The listing builds one solid part. Answer for the finished solid, in the listing's coordinates (mm). Face numbers are marked on the shaded views. A direction names the side the tool comes from. Round coordinates to 2 decimals unless told otherwise and drop trailing zeros. Order: outer loops, then holes, each group sorted by start corner. A loop starts at its lowest first (then second) coordinate and runs counter-clockwise, first axis right, second up. Notation, with made-up numbers: (-30.75, 9.5) - (-24.75, 9.5) arc R27 cw to (-24.75, 26.5) - close; hole circle Ø10 at (73, 26.5). An arc over 180 degrees is marked (long way). Write item = value, one per line.
Autodesk Fusion 360 part; units mm, degrees
sketch "Sketch1" plane through (0, 0, 0) normal (0, 0, 1) x (1, 0, 0)
  circle A0 centre (0, 0) radius 17.5
  dimension "d1" = 35
ref_plane "WorkPlane1" through (0, 0, 18) normal (0, 0, 1) x (1, 0, 0)
sketch "Sketch2" plane through (0, 0, 18) normal (0, 0, 1) x (1, 0, 0)
  circle A0 centre (0, 0) radius 17.5
  dimension "d3" = 35
ref_plane "WorkPlane2" through (0, 0, 9) normal (0, 0, 1) x (1, 0, 0)
sketch "Sketch3" plane through (0, 0, 9) normal (0, 0, 1) x (1, 0, 0)
  circle A0 centre (0, 0) radius 12.5
  dimension "d5" = 25
loft "Loft1" add profiles "Sketch2", "Sketch3" section 1 section 2
loft "Loft2" add profiles "Sketch1" section 1 section 2 face at (-3.3879, -0.621, 9)
extrude "Extrude1" add 1 faces at (4.4225, -5.9212, 18) along direction (0, 0, 1) blind 3
extrude "Extrude2" add 1 faces at (4.4225, -5.9212, 0) along direction (0, 0, -1) blind 3
sketch "Sketch4" plane through (0, 0, -3) normal (0, 0, -1) x (-1, 0, 0)
  circle A0 centre (0, 0) radius 17.5
  line L0 (2.8885, -3.049) -> (4.0848, 0.977)
  line L1 (4.0848, 0.977) -> (1.1962, 4.026)
  line L2 (1.1962, 4.026) -> (-2.8885, 3.049)
  line L3 (-2.8885, 3.049) -> (-4.0848, -0.977)
  line L4 (-4.0848, -0.977) -> (-1.1962, -4.026)
  line L5 (-1.1962, -4.026) -> (2.8885, -3.049)
  dimension "d10" = 4.2
extrude "Extrude3" cut sketch "Sketch4" against normal blind 15 contours L0 L1 L2 L3 L4 L5
sketch "Sketch5" plane through (0, 0, 21) normal (0, 0, 1) x (1, 0, 0)
  circle A0 centre (0, 0) radius 17.5
sketch "Sketch6" plane through (0, 0, 21) normal (0, 0, 1) x (1, 0, 0)
  circle A0 centre (0, 0) radius 7.5
  dimension "d13" = 15
extrude "Extrude4" cut sketch "Sketch6" against normal blind 7
sketch "Sketch7" plane through (0, 0, 21) normal (0, 0, 1) x (1, 0, 0)
  circle A0 centre (0, 0) radius 7.5
  dimension "d16" = 15
sketch "Sketch8" plane through (0, 0, 21) normal (0, 0, 1) x (1, 0, 0)
  circle A0 centre (0, 0) radius 2.5
  dimension "d17" = 5
extrude "Extrude5" cut sketch "Sketch8" against normal blind 9
equation "d4 = ( 18 / 2 ) * 1 mm"
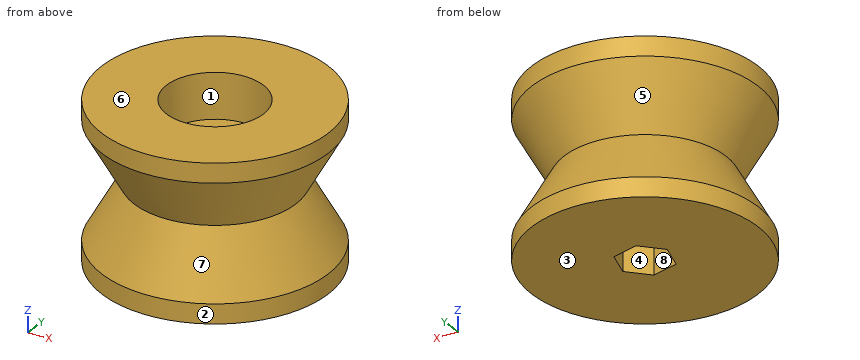
Q1. Section B-B on x = 0 is taken. Determine the outline of the cut face in (y, z), then the cut area to 3 significant figures.
Model answer:
outline = (-17.5, -3) - (-3.74, -3) - (-3.74, 12) - (-2.5, 12) - (-2.5, 14) - (-7.5, 14) - (-7.5, 21) - (-17.5, 21) - (-17.5, 18) - (-12.5, 9) - (-17.5, 0) - close; (2.5, 12) - (3.74, 12) - (3.74, -3) - (17.5, -3) - (17.5, 0) - (12.5, 9) - (17.5, 18) - (17.5, 21) - (7.5, 21) - (7.5, 14) - (2.5, 14) - close
area = 523 mm^2
Q2. Section C-C on z = -0.5 is taken. Determine the outline of the cut face in (x, y), then the cut area to 3 significant figures.
Model answer:
outline = circle Ø35 at (0, 0); hole (-4.08, 0.98) - (-2.89, -3.05) - (1.2, -4.03) - (4.08, -0.98) - (2.89, 3.05) - (-1.2, 4.03) - close
area = 916 mm^2
Q3. Find the intervals of material crossed by line 1 (Z direction, x = -5.5, y = -0.5); line 2 (Y direction, x = 0, z = 13.15); line 3 (X direction, y = 1, z = 12.5), in increasing order. Write a range as from..to.
Model answer:
line_1 = -3..14
line_2 = -14.81..-2.5, 2.5..14.81
line_3 = -14.41..-2.29, 2.29..14.41
Q4. For the marked faces 1, 2, 3, 4 and 5, determine the directions among +Z, -Z, +X, -X, +Y, -Y from which every point of the face is accessible in a straight line to the end or side of a thin tool.
Model answer:
face_1 = +Z
face_2 = +Z, -Z
face_3 = -Z, +X, -X, +Y, -Y
face_4 = -Z
face_5 = none
Q5. Flat-ended cylindrical pins translate along their axes: P1, Ø3, axis at x = 3.5, z = 1, coming from the +Y side; P2, Ø6.5, axis at x = 0, y = 0, coming from the -Z side; P3, Ø12, axis at x = 6, z = 4, coming from the -Y side. Find the tip coordinate at first contact, or state that the pin passes through.
Model answer:
P1 = 17.34
P2 = 12
P3 = -17.43
Q6. Determine the mould class of the marked faces 6, 7 and 8 for opening direction X: released by +X, released by -X, zero draft, split by the parting line, or undercut.
Model answer:
face_6 = zero draft
face_7 = split by the parting line
face_8 = undercut
Q7. Section D-D on z = 13.5 is taken. Determine the outline of the cut face in (x, y), then the cut area to 3 significant figures.
Model answer:
outline = circle Ø30 at (0, 0); hole circle Ø5 at (0, 0)
area = 687 mm^2
Q8. Section A-A on z = 6.75 is taken. Determine the outline of the cut face in (x, y).
Model answer:
outline = circle Ø27.5 at (0, 0); hole (-4.08, 0.98) - (-2.89, -3.05) - (1.2, -4.03) - (4.08, -0.98) - (2.89, 3.05) - (-1.2, 4.03) - close
